```python
from build123d import *

# Parameters (mm, degrees)
SKETCH1_W                                   = 220
SKETCH1_H                                   = 120
BOSS_EXTRUDE1_DEPTH                         = 14.5
CUT_EXTRUDE1_DEPTH                          = 26
FILLET1_R                                   = 1
FILLET2_R                                   = 10
CUT_EXTRUDE3_DEPTH                          = 3
CBORE_FOR_M4_CHEESE_HEAD_SCREW1_D           = 4.8
CBORE_FOR_M4_CHEESE_HEAD_SCREW1_CBORE_D     = 11.5
CBORE_FOR_M4_CHEESE_HEAD_SCREW1_CBORE_DEPTH = 20
FILLET3_R                                   = 5
SKETCH8_R                                   = 4.5
CUT_EXTRUDE4_DEPTH                          = 10
CUT_EXTRUDE5_REACH                          = 130.612
SKETCH9_R                                   = 10
M4_CLEARANCE_HOLE1_D                        = 4.3
CIRPATTERN1_COUNT                           = 4


with BuildPart() as part:
    # Sketch1 → Boss-Extrude1 (new, symmetric)
    with BuildSketch(Plane(origin=(0, 0, 0), x_dir=(0, 0, -1), z_dir=(1, 0, 0))):
        Rectangle(SKETCH1_W, SKETCH1_H)
    extrude(amount=BOSS_EXTRUDE1_DEPTH, both=True)

    # Sketch2 → Cut-Extrude1 (cut)
    with BuildSketch(Plane.ZY.offset(14.5)):
        Polygon((-87.25, 53.4), (87.25, 53.4), (87.25, 35.9), (103.4, 18.75), (103.4, -18.75), (87.25, -35.9), (87.25, -53.4), (-87.25, -53.4), (-87.25, -35.9), (-103.4, -18.75), (-103.4, 18.75), (-87.25, 35.9), align=None)
    extrude(amount=-CUT_EXTRUDE1_DEPTH, mode=Mode.SUBTRACT)

    # Fillet1
    fillet1_edges = [part.edges().sort_by_distance(p)[0] for p in [
        (-1.5, -18.75, 103.4),
        (-1.5, -53.4, 87.25),
        (-1.5, -53.4, -87.25),
        (-1.5, -18.75, -103.4),
        (-1.5, 18.75, -103.4),
        (-1.5, 53.4, -87.25),
        (-1.5, 53.4, 87.25),
        (-1.5, 18.75, 103.4),
    ]]
    fillet(fillet1_edges, radius=FILLET1_R)

    # Fillet2
    fillet2_edges = [part.edges().sort_by_distance(p)[0] for p in [
        (-1.5, -35.9, 87.25),
        (-1.5, -35.9, -87.25),
        (-1.5, 35.9, -87.25),
        (-1.5, 35.9, 87.25),
    ]]
    fillet(fillet2_edges, radius=FILLET2_R)

    # Sketch3 → Cut-Extrude3 (cut)
    with BuildSketch(Plane.ZY.offset(14.5)):
        with BuildLine():
            Line((92.05, 39.867350241), (92.05, 52.4))
            ThreePointArc((92.05, 52.4), (90.351219331, 56.501219331), (86.25, 58.2))
            Line((86.25, 58.2), (-86.25, 58.2))
            ThreePointArc((-86.25, 58.2), (-90.351219331, 56.501219331), (-92.05, 52.4))
            Line((-92.05, 52.4), (-92.05, 39.867350241))
            ThreePointArc((-92.05, 39.867350241), (-92.416498559, 37.949730931), (-93.464332239, 36.302421125))
            Line((-93.464332239, 36.302421125), (-106.62247558, 22.329532067))
            ThreePointArc((-106.62247558, 22.329532067), (-107.791213146, 20.492148053), (-108.2, 18.353264976))
            Line((-108.2, 18.353264976), (-108.2, -18.353264976))
            ThreePointArc((-108.2, -18.353264976), (-107.791213146, -20.492148053), (-106.62247558, -22.329532067))
            Line((-106.62247558, -22.329532067), (-93.464332239, -36.302421125))
            ThreePointArc((-93.464332239, -36.302421125), (-92.416498559, -37.949730931), (-92.05, -39.867350241))
            Line((-92.05, -39.867350241), (-92.05, -52.4))
            ThreePointArc((-92.05, -52.4), (-90.351219331, -56.501219331), (-86.25, -58.2))
            Line((-86.25, -58.2), (86.25, -58.2))
            ThreePointArc((86.25, -58.2), (90.351219331, -56.501219331), (92.05, -52.4))
            Line((92.05, -52.4), (92.05, -39.867350241))
            ThreePointArc((92.05, -39.867350241), (92.416498559, -37.949730931), (93.464332239, -36.302421125))
            Line((93.464332239, -36.302421125), (106.62247558, -22.329532067))
            ThreePointArc((106.62247558, -22.329532067), (107.791213146, -20.492148053), (108.2, -18.353264976))
            Line((108.2, -18.353264976), (108.2, 18.353264976))
            ThreePointArc((108.2, 18.353264976), (107.791213146, 20.492148053), (106.62247558, 22.329532067))
            Line((106.62247558, 22.329532067), (93.464332239, 36.302421125))
            ThreePointArc((93.464332239, 36.302421125), (92.416498559, 37.949730931), (92.05, 39.867350241))
        make_face()
        with BuildLine():
            ThreePointArc((-86.25, 55.4), (-88.371320344, 54.521320344), (-89.25, 52.4))
            Line((-89.25, 52.4), (-89.25, 39.867350241))
            ThreePointArc((-89.25, 39.867350241), (-89.813843937, 36.917166686), (-91.425895752, 34.382843909))
            Line((-91.425895752, 34.382843909), (-104.584039093, 20.409954851))
            ThreePointArc((-104.584039093, 20.409954851), (-105.188558524, 19.459583809), (-105.4, 18.353264976))
            Line((-105.4, 18.353264976), (-105.4, -18.353264976))
            ThreePointArc((-105.4, -18.353264976), (-105.188558524, -19.459583809), (-104.584039093, -20.409954851))
            Line((-104.584039093, -20.409954851), (-91.425895752, -34.382843909))
            ThreePointArc((-91.425895752, -34.382843909), (-89.813843937, -36.917166686), (-89.25, -39.867350241))
            Line((-89.25, -39.867350241), (-89.25, -52.4))
            ThreePointArc((-89.25, -52.4), (-88.371320344, -54.521320344), (-86.25, -55.4))
            Line((-86.25, -55.4), (86.25, -55.4))
            ThreePointArc((86.25, -55.4), (88.371320344, -54.521320344), (89.25, -52.4))
            Line((89.25, -52.4), (89.25, -39.867350241))
            ThreePointArc((89.25, -39.867350241), (89.813843937, -36.917166686), (91.425895752, -34.382843909))
            Line((91.425895752, -34.382843909), (104.584039093, -20.409954851))
            ThreePointArc((104.584039093, -20.409954851), (105.188558524, -19.459583809), (105.4, -18.353264976))
            Line((105.4, -18.353264976), (105.4, 18.353264976))
            ThreePointArc((105.4, 18.353264976), (105.188558524, 19.459583809), (104.584039093, 20.409954851))
            Line((104.584039093, 20.409954851), (91.425895752, 34.382843909))
            ThreePointArc((91.425895752, 34.382843909), (89.813843937, 36.917166686), (89.25, 39.867350241))
            Line((89.25, 39.867350241), (89.25, 52.4))
            ThreePointArc((89.25, 52.4), (88.371320344, 54.521320344), (86.25, 55.4))
            Line((86.25, 55.4), (-86.25, 55.4))
        make_face(mode=Mode.SUBTRACT)
    extrude(amount=-CUT_EXTRUDE3_DEPTH, mode=Mode.SUBTRACT)

    # CBORE for M4 Cheese Head Screw1 (through all)
    with Locations(Plane(origin=(14.5, 0, 0), x_dir=(0, 0, -1), z_dir=(1, 0, 0))):
        with Locations((99.75, 51), (-99.75, 51), (-99.75, -51), (99.75, -51)):
            CounterBoreHole(CBORE_FOR_M4_CHEESE_HEAD_SCREW1_D / 2, CBORE_FOR_M4_CHEESE_HEAD_SCREW1_CBORE_D / 2, CBORE_FOR_M4_CHEESE_HEAD_SCREW1_CBORE_DEPTH)

    # Fillet3
    fillet3_edges = [part.edges().sort_by_distance(p)[0] for p in [
        (0, 60, 110),
        (0, 60, -110),
        (0, -60, -110),
        (0, -60, 110),
    ]]
    fillet(fillet3_edges, radius=FILLET3_R)

    # Sketch8 → Cut-Extrude4 (cut)
    with BuildSketch(Plane.ZY.offset(14.5)):
        with Locations((99.75, 38.25)):
            Circle(SKETCH8_R)
        with Locations((99.75, -38.25)):
            Circle(SKETCH8_R)
        with Locations((-99.75, -38.25)):
            Circle(SKETCH8_R)
        with Locations((-99.75, 38.25)):
            Circle(SKETCH8_R)
    extrude(amount=-CUT_EXTRUDE4_DEPTH, mode=Mode.SUBTRACT)

    # Sketch9 → Cut-Extrude5 (cut, up to next)
    with BuildSketch(Plane(origin=(14.5, 0, 0), x_dir=(0, 0, -1), z_dir=(1, 0, 0)), mode=Mode.PRIVATE) as cut_extrude5_sk1:
        Circle(SKETCH9_R)
    cut_extrude5_tool1 = extrude(cut_extrude5_sk1.sketch, amount=-CUT_EXTRUDE5_REACH, mode=Mode.PRIVATE) & part.part
    add(cut_extrude5_tool1.solids().sort_by_distance((14.5, 0, 0))[0], mode=Mode.SUBTRACT)

    # M4 Clearance Hole1 (through all)
    with Locations(Plane(origin=(14.5, 0, 0), x_dir=(0, 0, -1), z_dir=(1, 0, 0))):
        with Locations((0, 20)):
            m4_clearance_hole1 = Hole(M4_CLEARANCE_HOLE1_D / 2)

    # CirPattern1: M4 Clearance Hole1 ×4 about axis
    cirpattern1_axis = Axis((0, 0, 0), (1, 0, 0))
    for i in range(1, CIRPATTERN1_COUNT):
        add(m4_clearance_hole1.rotate(cirpattern1_axis, i * 360 / CIRPATTERN1_COUNT), mode=Mode.SUBTRACT)


solid = part.part
```
The model under review builds one solid part; all positions refer to its coordinate system, in mm. A direction names the side the tool comes from. Round coordinates to 2 decimals unless told otherwise and drop trailing zeros. Loops run counter-clockwise (first coordinate to the right, second up) from the corner with the lowest first, then second, coordinate; pieces in that order, holes last. Notation, with made-up numbers: (65.25, 88.5) -> (115.25, 88.5) arc R12 ccw to (115.25, 96.5) -> close; hole circle Ø7 at (29.5, 32.25). An arc over 180 degrees is marked (long way). Answer in a Markdown table with one row per item.
1) Consider section B-B, the plane y = 0. Write out the cut boundary in (x, z), plus the area to 3 significant figures.
Taken from the geometry:
| item | result |
|---|---|
| outline | (-14.5, -110) -> (14.5, -110) -> (14.5, -22.15) -> (11.5, -22.15) -> (11.5, -103.4) -> (-14.5, -103.4) -> (-14.5, -105.4) -> (-11.5, -105.4) -> (-11.5, -108.2) -> (-14.5, -108.2) -> close; (-14.5, 103.4) -> (11.5, 103.4) -> (11.5, 22.15) -> (14.5, 22.15) -> (14.5, 110) -> (-14.5, 110) -> (-14.5, 108.2) -> (-11.5, 108.2) -> (-11.5, 105.4) -> (-14.5, 105.4) -> close; (11.5, -17.85) -> (14.5, -17.85) -> (14.5, -10) -> (11.5, -10) -> close; (11.5, 10) -> (14.5, 10) -> (14.5, 17.85) -> (11.5, 17.85) -> close |
| area | 901 mm² |
2) Consider section A-A, the plane z = -20. Write out the cut boundary in (x, y).
Taken from the geometry:
| item | result |
|---|---|
| outline | (-14.5, -60) -> (14.5, -60) -> (14.5, -2.15) -> (11.5, -2.15) -> (11.5, -53.4) -> (-14.5, -53.4) -> (-14.5, -55.4) -> (-11.5, -55.4) -> (-11.5, -58.2) -> (-14.5, -58.2) -> close; (-14.5, 53.4) -> (11.5, 53.4) -> (11.5, 2.15) -> (14.5, 2.15) -> (14.5, 60) -> (-14.5, 60) -> (-14.5, 58.2) -> (-11.5, 58.2) -> (-11.5, 55.4) -> (-14.5, 55.4) -> close |
3) Tool access review of faces 1 (the cylindrical face through (12.98, 17.9, -0.47)), 2 (the flat face through (-4.5, 38, 100)): name each direction out of +Z, -Z, +X, -X, +Y, -Y from which nothing blocks a thin tool from reaching the whole face with its end or side.
Taken from the geometry:
| item | result |
|---|---|
| face 1 | +X, -X |
| face 2 | -X |
4) Wall thickness on line 1 along Y through (x, z) = (13.05, 0); line 2 along Y through (x, z) = (0.5, -14.5); line 3 along Z through (x, y) = (3.5, 2.5): over which ranges is each line inside the solid? List them lowest first.
Taken from the geometry:
| item | result |
|---|---|
| line 1 | y = -60 to -22.15, -17.85 to -10, 10 to 17.85, 22.15 to 60 |
| line 2 | y = -60 to -53.4, 53.4 to 60 |
| line 3 | z = -110 to -103.4, 103.4 to 110 |
5) For pin 1 Ø3.5 at (y, z) = (49.5, -102) entering from +X; pin 2 Ø3 at (y, z) = (51, 99.75) entering from +X; pin 3 Ø2 at (y, z) = (-17, -32) entering from -X, all flat-tipped, find the tip position at first contact; note any pin that passes through.
Taken from the geometry:
| item | result |
|---|---|
| pin 1 | stops at x = -5.5 |
| pin 2 | passes through |
| pin 3 | stops at x = 11.5 |
6) Consider section C-C, the plane x = 1.25. Count the separate pieces of the cut face and the enclosed holes in it, plus the area to 3 significant figures.
Taken from the geometry:
| item | result |
|---|---|
| separate pieces | 1 |
| enclosed holes | 5 |
| area | 5,550 mm² |
7) Draft analysis for pull direction Z (two halves, no side actions). For faces 3 (the cylindrical face through (12.98, 0.47, 17.9)), 4 (the flat face through (0, -1, -110)), 5 (the flat face through (-14.5, 31.4, 98.3)), 6 (the flat face through (-2, 0, -103.4)), state which applies: pulls with the +Z half, pulls with the -Z half, needs draft (parallel to the pull), parting line crosses it, or undercut.
Taken from the geometry:
| item | result |
|---|---|
| face 3 | undercut |
| face 4 | pulls with the -Z half |
| face 5 | needs draft |
| face 6 | undercut |
